Autodesk Inventor part; units mm, degrees
ref_plane "Work Plane1" through (0, 753, 0) normal (0, 1, 0) x (1, 0, 0)
ref_plane "YZ Plane" through (0, 0, 0) normal (1, 0, 0) x (0, 1, 0)
ref_plane "XZ Plane" through (0, 0, 0) normal (0, 1, 0) x (-1, 0, 0)
sketch "Sketch1" plane through (0, 0, 0) normal (0, 1, 0) x (-1, 0, 0)
  line L0 (235, -200) -> (-235, -200)
  line L1 (-235, -200) -> (-235, 200)
  line L2 (-235, 200) -> (235, 200)
  line L3 (235, 200) -> (235, -200)
  line L4 (329, 0) -> (-329, 0)
  line L5 (0, -280) -> (0, 280)
  point P0 (0, 0)
  dimension "d0" = 470
  dimension "d1" = 400
extrude "Extrusion1" add sketch "Sketch1" along normal blind 20
sketch "Sketch2" plane through (0, 20, 0) normal (0, 1, 0) x (1, 0, 0)
  line L0 (-235, -200) -> (235, -200)
  line L1 (235, -200) -> (235, 200)
  line L2 (235, 200) -> (-235, 200)
  line L3 (-235, 200) -> (-235, -200)
  line L4 (-329, 0) -> (329, 0)
  line L5 (0, 280) -> (0, -280)
  circle A0 centre (0, 0) radius 20
  dimension "d4" = 40
extrude "Extrusion2" add sketch "Sketch2" along normal blind 125 contours A0 L4 L5 | L5 L4 A0 | A0 L5 L4 | L5 A0 L4
sketch "Sketch3" plane through (0, 145, 0) normal (0, 1, 0) x (1, 0, 0)
  line L0 (-151.5, 150.5) -> (151.5, 150.5)
  line L1 (151.5, 150.5) -> (151.5, -150.5)
  line L2 (151.5, -150.5) -> (-151.5, -150.5)
  line L3 (-151.5, -150.5) -> (-151.5, 150.5)
  line L4 (-329, 0) -> (329, 0)
  line L5 (0, 280) -> (0, -280)
  point P0 (0, 0)
  dimension "d7" = 303
  dimension "d8" = 301
extrude "Extrusion3" add sketch "Sketch3" along normal blind 8
ref_plane "Work Plane1" through (0, 753, 0) normal (0, 1, 0) x (1, 0, 0)
sketch "Sketch4" plane through (0, 753, 0) normal (0, 1, 0) x (1, 0, 0)
  line L0 (-235, 10) -> (235, 10)
  line L1 (235, 10) -> (235, -10)
  line L2 (235, -10) -> (-235, -10)
  line L3 (-235, -10) -> (-235, 10)
  circle A0 centre (0, 0) radius 20
  line L4 (-235, -200) -> (235, -200)
  line L5 (235, -200) -> (235, 200)
  line L6 (235, 200) -> (-235, 200)
  line L7 (-235, 200) -> (-235, -200)
  line L8 (-329, 0) -> (329, 0)
  line L9 (0, 280) -> (0, -280)
  dimension "d12" = 20
extrude "Extrusion4" add sketch "Sketch4" along normal blind 20 contours L0 A0 L8 L3 | L0 L9 L8 A0 | L8 A0 L2 L3 | L0 A0 L8 L9 | L8 L9 L2 A0 | L0 L1 L8 A0 | L8 A0 L2 L9 | L8 L1 L2 A0
sketch "Sketch5" plane through (235, 0, 200) normal (1, 0, 0) x (0, 0, -1)
  line L0 (190, 753) -> (210, 753)
  line L1 (210, 753) -> (210, 773)
  line L2 (190, 773) -> (210, 773)
  line L3 (190, 753) -> (190, 773)
  line L4 (0, 0) -> (400, 0)
  line L5 (0, 20) -> (400, 20)
  line L6 (0, 0) -> (0, 20)
  line L7 (400, 0) -> (400, 20)
  line L8 (0, 0) -> (400, 0)
  line L9 (400, 0) -> (400, 20)
  line L10 (0, 20) -> (400, 20)
  line L11 (0, 0) -> (0, 20)
  line L12 (160.0551, 773) -> (239.9449, 773)
  line L13 (0, 20) -> (160.0551, 773)
  line L14 (200, -184.6) -> (200, 1107.6)
  line L15 (400, 20) -> (239.9449, 773)
  line L16 (190, 773) -> (210, 773)
  line L17 (0, 20) -> (51.117, 20)
  line L18 (348.883, 20) -> (400, 20)
  line L19 (348.883, 20) -> (200, 720.4393)
  line L20 (51.117, 20) -> (200, 720.4393)
  line L21 (150, 690) -> (250, 690) construction
  line L22 (250, 690) -> (250, 563) construction
  line L23 (250, 563) -> (150, 563) construction
  line L24 (150, 563) -> (150, 690) construction
  point P0 (200, 0)
  point P1 (183.5455, 773)
  point P2 (216.4545, 773)
  dimension "d16" = 78
  dimension "d18" = 78
  dimension "d26" = 50
  dimension "d27" = 100
  dimension "d28" = 127
  dimension "d29" = 670
extrude "Extrusion5" add sketch "Sketch5" against normal blind 20 contours L3 L2 L14 L0 | L0 L14 L20 L5 L13 L12 L3 | L14 L2 L1 L0 | L0 L1 L12 L15 L5 L19 L14
sketch "Sketch6" plane through (-235, 753, -10) normal (-1, 0, 0) x (0, 0, 1)
  line L0 (-40, -60) -> (60, -60) construction
  line L1 (60, -60) -> (60, -188) construction
  line L2 (60, -188) -> (-40, -188) construction
  line L3 (-40, -188) -> (-40, -60) construction
  line L4 (10, -925.1189) -> (10, 279.7131)
  line L5 (0, 0) -> (20, 0)
  line L6 (20, 0) -> (20, 20)
  line L7 (0, 20) -> (20, 20)
  line L8 (0, 0) -> (0, 20)
  line L9 (20, 0) -> (20, 20)
  line L10 (0, 0) -> (20, 0)
  line L11 (0, 20) -> (0, 0)
  line L12 (0, 20) -> (-29.9449, 20)
  line L13 (-29.9449, 20) -> (-190, -733)
  line L14 (-138.883, -733) -> (-190, -733)
  line L15 (210, -733) -> (49.9449, 20)
  line L16 (49.9449, 20) -> (20, 20)
  line L17 (-29.9449, 20) -> (-190, -733)
  line L18 (-190, -733) -> (-29.9449, 20)
  line L19 (-29.9449, 20) -> (49.9449, 20)
  line L20 (210, -733) -> (49.9449, 20)
  line L21 (159.2287, -733) -> (210, -733)
  line L22 (159.2287, -733) -> (39.7909, 107.5943)
  line L23 (-138.883, -733) -> (39.7909, 107.5943)
  line L24 (39.7909, 107.5943) -> (-138.883, -733)
  line L25 (-138.883, -733) -> (-190, -733)
  line L26 (-138.883, -733) -> (10, -32.5607)
  line L27 (10, -32.5607) -> (158.883, -733)
  line L28 (210, -733) -> (158.883, -733)
  point P0 (10, -753)
  point P1 (0, 20)
  dimension "d21" = 100
  dimension "d22" = 128
  dimension "d23" = 60
extrude "Extrusion6" add sketch "Sketch6" against normal blind 20 contours L23 L14 L13 L12 L8 L5 L4 | L4 L5 L23 | L23 L5 L6 L16 L15 L22 L28 L27 | L6 L16 L23 | L22 L15 L21
properties part number "Estructura AA"
Verification items for the finished model (mm, model axes). A direction names the side the tool comes from. Give positions to 0.01 mm unless a question says otherwise; leave off trailing zeros. Order: outer loops, then holes, each group sorted by start corner. A loop starts at its lowest first (then second) coordinate and runs counter-clockwise, first axis right, second up. Notation, with made-up numbers: (82, 49.5) -> (91, 49.5) arc R11 cw to (91, 69.5) -> close; hole circle Ø7 at (-1.5, 50). An arc over 180 degrees is marked (long way). Use a Markdown table: item, result.
1) Section check B-B, the plane y = 405. Record the boundary of the cut face in (x, z).
Results:
| item | result |
|---|---|
| outline | (-235, -118.17) -> (-215, -118.17) -> (-215, -67.05) -> (-235, -67.05) -> close; (-235, 67.05) -> (-215, 67.05) -> (-215, 118.17) -> (-235, 118.17) -> close; (215, -118.17) -> (235, -118.17) -> (235, -67.05) -> (215, -67.05) -> close; (215, 67.05) -> (235, 67.05) -> (235, 118.17) -> (215, 118.17) -> close |
2) Section check C-C, the plane z = -122. Record the boundary of the cut face in (x, y), then the cut area to 3 significant figures.
Results:
| item | result |
|---|---|
| outline | (-235, 0) -> (235, 0) -> (235, 20) -> (-235, 20) -> close; (-235, 146.47) -> (-215, 146.47) -> (-215, 386.96) -> (-235, 386.96) -> close; (-151.5, 145) -> (151.5, 145) -> (151.5, 153) -> (-151.5, 153) -> close; (215, 146.47) -> (235, 146.47) -> (235, 386.96) -> (215, 386.96) -> close |
| area | 21,400 mm² |
3) Section check D-D, the plane x = 203.5. Record the boundary of the cut face in (y, z).
Results:
| item | result |
|---|---|
| outline | (0, -200) -> (20, -200) -> (20, 200) -> (0, 200) -> close; (753, -10) -> (773, -10) -> (773, 10) -> (753, 10) -> close |
4) Depth check by flat-ended pin: pin 1 Ø1.5 at (x, z) = (-89, 66) entering from +Y; pin 2 Ø5 at (x, z) = (171.5, -158) entering from +Y; pin 3 Ø16 at (x, y) = (50.5, 760) entering from +Z. Enter the tip coordinate at first touch or a pass-through.
Results:
| item | result |
|---|---|
| pin 1 | y = 153 |
| pin 2 | y = 20 |
| pin 3 | z = 10 |
5) Tool access check on faces 1 (the flat face through (235, 385, 73)), 2 (the flat face through (3, 763, 10)), 3 (the flat face through (-3, 753, 0)). Record the directions out of +Z, -Z, +X, -X, +Y, -Y that give a thin tool (end or side, any length) a straight path to the whole face; none if there is none.
Results:
| item | result |
|---|---|
| face 1 | +Z, -Z, +X, +Y, -Y |
| face 2 | +Z, +Y |
| face 3 | +Z, -Z |
6) Material ranges on probe 1 along X at (y, z) = (698, -53.5); probe 2 along Y at (x, z) = (-97, -21); probe 3 along Y at (x, z) = (187.5, 91.5), recorded low to high.
Results:
| item | result |
|---|---|
| probe 1 | -235 to -215, 215 to 235 |
| probe 2 | 0 to 20, 145 to 153 |
| probe 3 | 0 to 20 |
7) Section check A-A, the plane x = 0. Record the boundary of the cut face in (y, z), then the cut area to 3 significant figures.
Results:
| item | result |
|---|---|
| outline | (0, -200) -> (20, -200) -> (20, -20) -> (145, -20) -> (145, -150.5) -> (153, -150.5) -> (153, 150.5) -> (145, 150.5) -> (145, 20) -> (20, 20) -> (20, 200) -> (0, 200) -> close; (753, -10) -> (773, -10) -> (773, 10) -> (753, 10) -> close |
| area | 15,800 mm² |
8) Mould release check, pull along X, two halves, no side actions. Record for faces 4 (the flat face through (-235, 385, -73)), 5 (the flat face through (-225.14, 375.12, 73.4)), 6 (the flat face through (-3, 763, -10)): pulls with the +X half, pulls with the -X half, needs draft (parallel to the pull), parting line crosses it, or undercut.
Results:
| item | result |
|---|---|
| face 4 | pulls with the -X half |
| face 5 | needs draft |
| face 6 | undercut |
